```python
from build123d import *

# Parameters (mm, degrees)
SKETCH_1_R          = 1.1
EXTRUDE_1_DEPTH     = 2
SKETCH_2_W          = 9
SKETCH_2_H          = 3.8
CUT_EXTRUDE_1_DEPTH = 11.198039027
FILLET_1_R          = 2
FILLET_2_R          = 1


with BuildPart() as part:
    # 草图1 → 凸台-拉伸1 (new body)
    with BuildSketch(Plane(origin=(0, 0, 0), x_dir=(1, 0, 0), z_dir=(0, 1, 0))):
        Polygon((-8, 6), (-8, -6), (8, -6), (8, 6), (2.25, 6), (2.25, -3.5), (-2.25, -3.5), (-2.25, 6), align=None)
        with Locations(Location((-6, -4, 0), (0, 0, 270))):
            Circle(SKETCH_1_R, mode=Mode.SUBTRACT)
        with Locations(Location((6, -4, 0), (0, 0, 270))):
            Circle(SKETCH_1_R, mode=Mode.SUBTRACT)
        with Locations(Location((-6, 4, 0), (0, 0, 270))):
            Circle(SKETCH_1_R, mode=Mode.SUBTRACT)
        with Locations(Location((6, 4, 0), (0, 0, 270))):
            Circle(SKETCH_1_R, mode=Mode.SUBTRACT)
    extrude(amount=EXTRUDE_1_DEPTH)

    # 草图2 → 切除-拉伸1 (cut, through all)
    with BuildSketch(Plane(origin=(0, 2, 0), x_dir=(1, 0, 0), z_dir=(0, 1, 0))):
        Rectangle(SKETCH_2_W, SKETCH_2_H)
    extrude(amount=-CUT_EXTRUDE_1_DEPTH, mode=Mode.SUBTRACT)

    # 圆角1
    fillet_1_edges = [part.edges().sort_by_distance(p)[0] for p in [
        (8, 1, -6),
        (8, 1, 6),
        (-8, 1, 6),
        (-8, 1, -6),
    ]]
    fillet(fillet_1_edges, radius=FILLET_1_R)

    # 圆角2
    fillet_2_edges = [part.edges().sort_by_distance(p)[0] for p in [
        (-2.25, 1, 3.5),
        (2.25, 1, 3.5),
        (-4.5, 1, -1.9),
        (4.5, 1, -1.9),
        (4.5, 1, 1.9),
        (-4.5, 1, 1.9),
    ]]
    fillet(fillet_2_edges, radius=FILLET_2_R)


solid = part.part
```
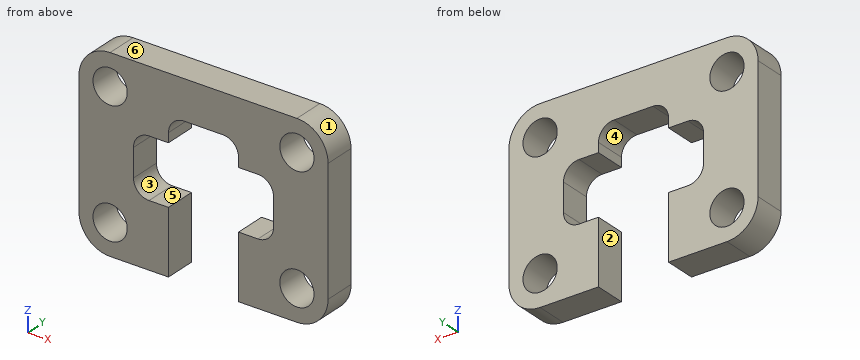
Geometry check sheet. Reference: the model listing, model coordinates, mm. Face numbers are marked on the shaded views. A direction names the side the tool comes from. Coordinates: 2 decimals unless noted, no trailing zeros. Write each loop counter-clockwise with the first axis right and the second up, starting at its lowest first coordinate (ties: lowest second). Pieces come first, ordered by that corner, then holes. Notation, with made-up numbers: M -10,88.5 L 14,88.5 A8 ccw 14,100.5 Z; hole C 64.5,-30.75 d9. An arc over 180 degrees is marked long. Answer as a JSON object with one key per item and string values.
1. Draft check along Z on the marked faces 1, 2 and 3. Enter one of: released by +Z, released by -Z, zero draft, split by the parting line, or undercut.
Answers below:
{"face 1": "released by +Z", "face 2": "zero draft", "face 3": "undercut"}
2. Section check C-C, the plane x = -4. Enter the section's corners in (y, z).
Answers below:
{"outline": "M 0,-6 L 2,-6 L 2,-1.77 L 0,-1.77 Z; M 0,1.77 L 2,1.77 L 2,6 L 0,6 Z"}
3. Scan lines: L1, parallel to X at y = 0.75, z = -4; L2, parallel to X at y = 1, z = 4; L3, parallel to X at y = 1.2, z = 0.25. Record each from-to range of solid material in increasing order.
Answers below:
{"L1": "x = -8 to -7.1, -4.9 to -2.25, 2.25 to 4.9, 7.1 to 8", "L2": "x = -8 to -7.1, -4.9 to 4.9, 7.1 to 8", "L3": "x = -8 to -4.5, 4.5 to 8"}
4. Section check B-B, the plane y = 1.2. Give the number of separate pieces and of enclosed holes in the cut face, plus the area to 3 significant figures.
Answers below:
{"separate pieces": "1", "enclosed holes": "4", "area": "115 mm²"}
5. Section check A-A, the plane z = -1.5. Enter the section's corners in (x, y), plus the area to 3 significant figures.
Answers below:
{"outline": "M -8,0 L -4.3,0 L -4.3,2 L -8,2 Z; M 4.3,0 L 8,0 L 8,2 L 4.3,2 Z", "area": "14.8 mm²"}
6. Go/stop test with a flat-tipped pin: pin 1 Ø1.8 at (x, z) = (-6, 4) entering from -Y. Record where the tip stops, or that it passes through.
Answers below:
{"pin 1": "passes through"}
7. Section check D-D, the plane x = 1.75. Enter the section's corners in (y, z), plus the area to 3 significant figures.
Answers below:
{"outline": "M 0,3.37 L 2,3.37 L 2,6 L 0,6 Z", "area": "5.27 mm²"}
8. Tool access check on the marked faces 4, 5 and 6. Record the directions out of +Z, -Z, +X, -X, +Y, -Y that give a thin tool (end or side, any length) a straight path to the whole face; none if there is none.
Answers below:
{"face 4": "-Z, +Y, -Y", "face 5": "+Y, -Y", "face 6": "+Z, +X, -X, +Y, -Y"}
